Input: dimensioned drawing with shaded views. Units: mm. Origin: part minimum x, y, z. A direction names the side the tool comes from. Coordinates: 2 decimals unless noted, no trailing zeros. Order: outer loops, then holes, each group sorted by start corner. A loop starts at its lowest first (then second) coordinate and runs counter-clockwise, first axis right, second up. Notation, with made-up numbers: M 62,86.5 L 83,86.5 A28 cw 83,115.5 Z; hole C -26.5,-16.75 d5. An arc over 180 degrees is marked long. Write item = value, one per line.
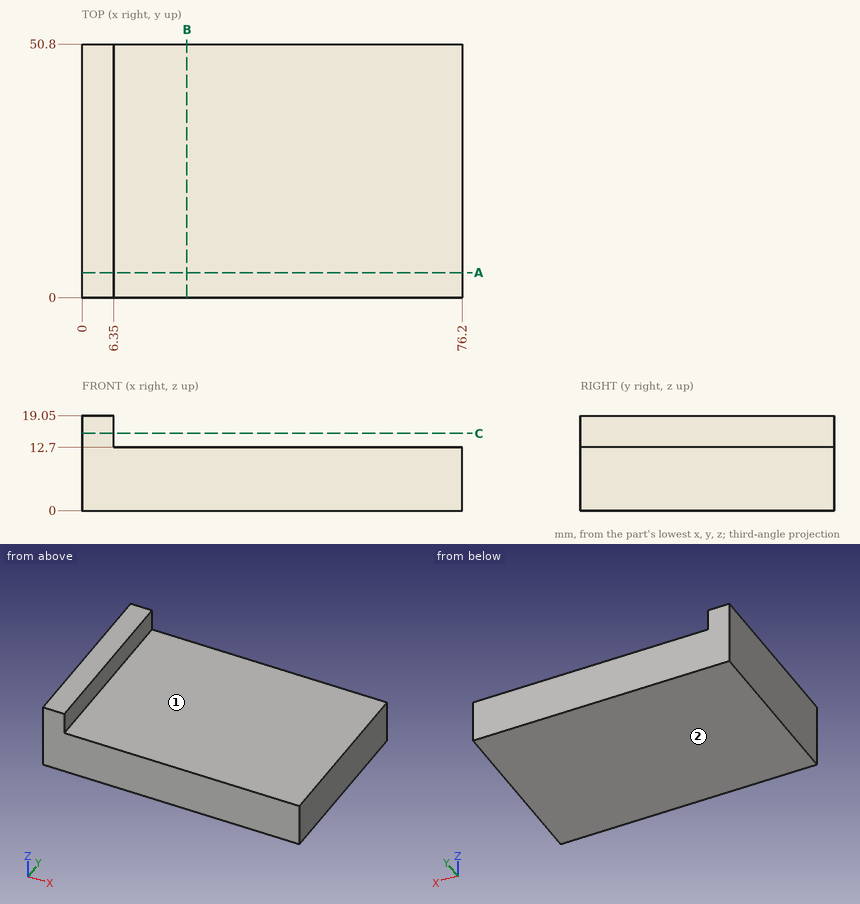
1) Section A-A, the plane y = 5. Return loops of the section in (x, z).
Numbers:
outline = M 0,0 L 76.2,0 L 76.2,12.7 L 6.35,12.7 L 6.35,19.05 L 0,19.05 Z
2) Set-up query: the marked faces 1 and 2. Return all of +Z, -Z, +X, -X, +Y, -Y with unobstructed straight access to the full face (end or side cutting, diameter ignored); none if empty.
Numbers:
face_1 = +Z, +X, +Y, -Y
face_2 = -Z, +X, -X, +Y, -Y
3) Section B-B, the plane x = 21. Return loops of the section in (y, z).
Numbers:
outline = M 0,0 L 50.8,0 L 50.8,12.7 L 0,12.7 Z
4) Line query: L1, parallel to Z at x = 28.5, y = 18; L2, parallel to X at y = 37.5, z = 14. Output: solid intervals per line, ascending.
Numbers:
L1 = 0 to 12.7
L2 = 0 to 6.35
5) Pin query (flat end, axial travel): pin 1 (4 mm diameter, centred on x = 45.5, y = 37.5, fed in from +Z). Return the tip coordinate at first contact, or that it passes through.
Numbers:
pin_1 = 12.7
6) Section C-C, the plane z = 15.5. Return loops of the section in (x, y), and give its area (3 significant figures).
Numbers:
outline = M 0,0 L 6.35,0 L 6.35,50.8 L 0,50.8 Z
area = 323 mm²
